Autodesk Inventor part; units mm, degrees
ref_plane "YZ Plane" through (0, 0, 0) normal (1, 0, 0) x (0, 1, 0)
ref_plane "XZ Plane" through (0, 0, 0) normal (0, 1, 0) x (-1, 0, 0)
ref_plane "XY Plane" through (0, 0, 0) normal (0, 0, 1) x (1, 0, 0)
sketch "Sketch1" plane through (0, 0, 0) normal (1, 0, 0) x (0, 1, 0)
  line L0 (-55, 110) -> (55, 110)
  line L1 (55, 110) -> (55, -110)
  line L2 (55, -110) -> (-55, -110)
  line L3 (-55, -110) -> (-55, 110)
  line L4 (-55, 110) -> (55, -110) construction
  line L5 (55, 110) -> (-55, -110) construction
  circle A0 centre (-15, 32.5) radius 4.1
  circle A1 centre (-15, -32.5) radius 4.1
  circle A2 centre (-15, 0) radius 5
  line L6 (-15, 32.5) -> (-15, -32.5) construction
  line L7 (48, -103) -> (48, 103)
  line L8 (48, 103) -> (-48, 103)
  line L9 (-48, 103) -> (-48, -103)
  line L10 (-48, -103) -> (48, -103)
  point P0 (0, 0)
  dimension "d0" = 65
  dimension "d1" = 8.2
  dimension "d2" = 220
  dimension "d3" = 110
  dimension "d4" = 7
  dimension "d35" = 10
  dimension "d36" = 15
extrude "Extrusion1" add sketch "Sketch1" along normal blind 8 contours L0 L1 L2 L3 | A0 | A1 | L10 L9 L8 L7
sketch "Sketch2" plane through (8, 0, 0) normal (1, 0, 0) x (0, 0, -1)
  line L0 (110, -55) -> (110, 55)
  line L1 (110, 55) -> (-110, 55)
  line L2 (-110, 55) -> (-110, -55)
  line L3 (-110, -55) -> (110, -55)
  line L4 (-33.234, -33.234) -> (33.234, -33.234) construction
  line L5 (33.234, -33.234) -> (33.234, 33.234) construction
  line L6 (33.234, 33.234) -> (-33.234, 33.234) construction
  line L7 (-33.234, 33.234) -> (-33.234, -33.234) construction
  line L8 (-33.234, -33.234) -> (33.234, 33.234) construction
  line L9 (33.234, -33.234) -> (-33.234, 33.234) construction
  circle A0 centre (0, 0) radius 47 construction
  circle A1 centre (33.234, 33.234) radius 2.75
  circle A2 centre (-33.234, 33.234) radius 2.75
  circle A3 centre (0, 0) radius 47 construction
  circle A4 centre (-33.234, -33.234) radius 2.75
  circle A5 centre (0, 0) radius 47 construction
  circle A6 centre (33.234, -33.234) radius 2.75
  circle A7 centre (0, 0) radius 47 construction
  point P0 (0, 0)
  point P1 (0, 0)
  dimension "d12" = 94
  dimension "d13" = 5.5
  dimension "d16" = 360
extrude "Extrusion3" cut sketch "Sketch2" against normal through all contours A1 | A2 | A4 | A6
sketch "Sketch3" plane through (0, 0, 0) normal (-1, 0, 0) x (0, 0, 1)
  circle A0 centre (33.234, -33.234) radius 2.75
  circle A1 centre (33.234, 33.234) radius 2.75
  circle A2 centre (-33.234, -33.234) radius 2.75
  circle A3 centre (-33.234, 33.234) radius 2.75
  circle A4 centre (0, -15) radius 5
  circle A5 centre (-33.234, 33.234) radius 4.5
  circle A6 centre (33.234, 33.234) radius 2.75
  circle A7 centre (33.234, 33.234) radius 4.5
  circle A8 centre (-33.234, -33.234) radius 4.5
  circle A9 centre (33.234, -33.234) radius 4.5
  point P0 (0, 0)
  dimension "d20" = 9
extrude "Extrusion4" cut sketch "Sketch3" against normal blind 3 contours A0 | A1 | A2 | A3 | A5 | A7 | A8 | A9
sketch "Sketch4" plane through (8, 0, 0) normal (1, 0, 0) x (0, 0, -1)
  circle A0 centre (-33.234, -33.234) radius 2.75
  circle A1 centre (-33.234, 33.234) radius 2.75
  circle A2 centre (33.234, -33.234) radius 2.75
  circle A3 centre (33.234, 33.234) radius 2.75
  line L0 (110, -55) -> (110, 55)
  line L1 (110, 55) -> (-110, 55)
  line L2 (-110, 55) -> (-110, -55)
  line L3 (-110, -55) -> (110, -55)
  circle A4 centre (0, -15) radius 5
  circle A5 centre (0, -15) radius 10.3
  point P0 (0, 0)
  dimension "d24" = 20.6
extrude "Extrusion5" cut sketch "Sketch4" against normal through all contours A4 | A5
sketch "Sketch7" plane through (0, 0, 0) normal (-1, 0, 0) x (0, 0, 1)
  line L0 (-50, -45.3941) -> (50, -45.3941)
  line L1 (50, -45.3941) -> (50, 4.6059)
  line L2 (50, 4.6059) -> (-50, 4.6059)
  line L3 (-50, 4.6059) -> (-50, -45.3941)
  circle A0 centre (-32.5, -15) radius 4.1
  circle A1 centre (32.5, -15) radius 4.1
  line L4 (-110, -55) -> (-110, 55)
  line L5 (-110, 55) -> (110, 55)
  line L6 (110, 55) -> (110, -55)
  line L7 (110, -55) -> (-110, -55)
  point P0 (0, 4.6059)
  point P1 (0, 4.6059)
  point P2 (0, -15)
  dimension "d37" = 50
  dimension "d38" = 100
extrude "Extrusion8" cut sketch "Sketch7" against normal through all
chamfer "Chamfer3" distance 15 angle 45 2 edges at (4, -45.3941, -50) (4, -45.3941, 50)
chamfer "Chamfer4" distance 8 angle 45 2 edges at (4, 4.6059, -50) (4, 4.6059, 50)
sketch "Sketch8" plane through (0, 0, 0) normal (-1, 0, 0) x (0, 0, 1)
  circle A0 centre (-32.5, -15) radius 4.1
  circle A1 centre (32.5, -15) radius 4.1
  circle A2 centre (-32.5, -15) radius 6
  circle A3 centre (32.5, -15) radius 6
  point P0 (0, 0)
  dimension "d47" = 12
extrude "Extrusion9" add sketch "Sketch8" along normal blind 5
sketch "Sketch9" plane through (8, 0, 0) normal (1, 0, 0) x (0, 0, -1)
  circle A0 centre (-32.5, -15) radius 4.1
  circle A1 centre (32.5, -15) radius 4.1
  point P0 (0, 0)
extrude "Extrusion10" add sketch "Sketch9" against normal blind 4
sketch "Sketch10" plane through (0, 0, 0) normal (-1, 0, 0) x (0, 0, 1)
  circle A0 centre (0, -15) radius 10.3
  circle A1 centre (-15, -15) radius 2.75
  circle A2 centre (15, -15) radius 2.75
  line L0 (-15, -15) -> (15, -15) construction
  point P0 (0, 0)
  dimension "d52" = 30
  dimension "d53" = 5.5
extrude "Extrusion11" cut sketch "Sketch10" against normal through all contours A1 | A2
fillet "Fillet2" radius 2 2 edges at (0, -15, -38.5) (0, -15, 26.5)
properties part number "CAJA" material "Steel, Mild, Welded"
Design review of the part built by this model. Coordinates are the model's own, in mm. A direction names the side the tool comes from. Give positions to 0.01 mm unless a question says otherwise; leave off trailing zeros. Order: outer loops, then holes, each group sorted by start corner. A loop starts at its lowest first (then second) coordinate and runs counter-clockwise, first axis right, second up. Notation, with made-up numbers: (49, 22) -> (90, 22) arc R21 ccw to (90, 45) -> close; hole circle Ø1 at (75.25, 24). An arc over 180 degrees is marked (long way). Write each question's results on one line, items separated by ' | '. Start each with the question number.
Q1. Mouldability with a two-part tool opening along Y and no side actions: class faces 3 (the cylindrical face through (3.944, -14.879, 12.253)), 4 (the flat face through (4.056, 0.662, -45.944)), 5 (the flat face through (3, -36.2, 33.2)), 6 (the flat face through (-5, -19, 34)) as +Y half, -Y half, draft (parallel to the pull), parting line (faces both ways), or undercut.
Q2. For pin 1 (11.5 mm diameter, centred on y = -33.234, z = 33.234, fed in from -X); pin 2 (5 mm diameter, centred on y = -15, z = -32.5, fed in from -X); pin 3 (7 mm diameter, centred on y = -33.234, z = -33.234, fed in from +X); pin 4 (4.5 mm diameter, centred on y = -34, z = -34.5, fed in from -X), all flat-tipped, find the tip position at first contact; note any pin that passes through.
Q3. Machinability: for faces 1 (the cylindrical face through (-3.479, -15.264, 26.506)), 2 (the cylindrical face through (4.056, -25.055, 2.233)), which of the approach directions +Z, -Z, +X, -X, +Y, -Y give a long, thin tool a straight path to every point of the face, cutting with its end or side? Answer none if there is none.
Q4. Add section D-D on z = 0. Give the boundary of the cut face in (x, y), and give its area (3 significant figures).
Q5. Add section A-A on z = 15. Give the boundary of the cut face in (x, y), and give its area (3 significant figures).
Q6. Add section C-C on x = -3. Give the boundary of the cut face in (y, z), and give its area (3 significant figures).
Q7. Wall thickness on L1, parallel to Y at x = -2, z = -32.5; L2, parallel to Z at x = 7.25, y = -33.5; L3, parallel to Y at x = 0.25, z = 0.5: over which ranges is each line inside the solid? List them lowest first. Write a range as from..to.
Q8. Add section B-B on x = 1.75. Give the boundary of the cut face in (y, z), and give its area (3 significant figures).
Found:
1) face 3: undercut | face 4: +Y half | face 5: undercut | face 6: draft
2) pin 1: stops at x = 0 | pin 2: stops at x = 4 | pin 3: stops at x = 8 | pin 4: stops at x = 3
3) face 1: -X | face 2: +X, -X
4) outline: (0, -45.39) -> (8, -45.39) -> (8, -25.3) -> (0, -25.3) -> close; (0, -4.7) -> (8, -4.7) -> (8, 4.61) -> (0, 4.61) -> close | area: 235 mm2
5) outline: (0, -45.39) -> (8, -45.39) -> (8, -17.75) -> (0, -17.75) -> close; (0, -12.25) -> (8, -12.25) -> (8, 4.61) -> (0, 4.61) -> close | area: 356 mm2
6) outline: circle Ø12 at (-15, -32.5); circle Ø12 at (-15, 32.5); hole circle Ø8.2 at (-15, -32.5); hole circle Ø8.2 at (-15, 32.5) | area: 121 mm2
7) L1: y = -21..-19.1, -10.9..-9 | L2: z = -46.89..-35.97, -30.5..30.5, 35.97..46.89 | L3: y = -45.39..-25.29, -4.71..4.61
8) outline: (-45.39, -35) -> (-30.39, -50) -> (-3.39, -50) -> (4.61, -42) -> (4.61, 42) -> (-3.39, 50) -> (-30.39, 50) -> (-45.39, 35) -> close; hole circle Ø9 at (-33.23, -33.23); hole circle Ø9 at (-33.23, 33.23); hole circle Ø20.6 at (-15, 0); hole circle Ø8.2 at (-15, -32.5); hole circle Ø8.2 at (-15, 32.5); hole circle Ø5.5 at (-15, -15); hole circle Ø5.5 at (-15, 15) | area: 4,100 mm2
